The model under review builds one solid part; all positions refer to its coordinate system, in mm. A direction names the side the tool comes from. Coordinates: 2 decimals unless noted, no trailing zeros. Order: outer loops, then holes, each group sorted by start corner. A loop starts at its lowest first (then second) coordinate and runs counter-clockwise, first axis right, second up.
```python
from build123d import *

# Parameters (mm, degrees)
SKETCH1_W               = 28
SKETCH1_H               = 27
BOSS_EXTRUDE1_DEPTH     = 1.4
SKETCH2_R               = 1.55
CUT_EXTRUDE1_DEPTH      = 20.498974332
FILLET1_R               = 2
FILLET2_R               = 2
BOSS_EXTRUDE2_DEPTH     = 20
SKETCH5_W               = 14.5
SKETCH5_H               = 1
BOSS_EXTRUDE3_DEPTH     = 20
FILLET3_R               = 4
FILLET4_R               = 3
CUT_EXTRUDE2_DEPTH      = 32.957002439
CUT_EXTRUDE2_DEPTH_BACK = 32.957002439
FILLET6_R               = 2
FILLET7_R               = 3
SKETCH7_R               = 1.25
BOSS_EXTRUDE4_DEPTH     = 14.5
SKETCH8_R               = 6.5
BOSS_EXTRUDE5_DEPTH     = 5.5
FILLET8_R               = 1


with BuildPart() as part:
    # Sketch1 → Boss-Extrude1 (new body)
    with BuildSketch(Plane(origin=(0, 0, 0), x_dir=(1, 0, 0), z_dir=(0, 1, 0))):
        Rectangle(SKETCH1_W, SKETCH1_H)
    extrude(amount=BOSS_EXTRUDE1_DEPTH)

    # Sketch2 → Cut-Extrude1 (cut, through all)
    with BuildSketch(Plane(origin=(0, 1.4, 0), x_dir=(1, 0, 0), z_dir=(0, 1, 0))):
        with Locations(Location((-11, 10, 0), (0, 0, 270))):
            Circle(SKETCH2_R)
        with Locations(Location((-11, -10, 0), (0, 0, 270))):
            Circle(SKETCH2_R)
        with Locations(Location((11, -10, 0), (0, 0, 270))):
            Circle(SKETCH2_R)
        with Locations(Location((11, 10, 0), (0, 0, 270))):
            Circle(SKETCH2_R)
    extrude(amount=-CUT_EXTRUDE1_DEPTH, mode=Mode.SUBTRACT)

    # Fillet1
    fillet1_edges = [part.edges().sort_by_distance(p)[0] for p in [
        (-14, 0.7, -13.5),
        (14, 0.7, -13.5),
        (14, 0.7, 13.5),
        (-14, 0.7, 13.5),
    ]]
    fillet(fillet1_edges, radius=FILLET1_R)

    # Sketch3 → Revolve1 (revolve)
    with BuildSketch(Plane(origin=(0, 0, 0), x_dir=(0, 0, -1), z_dir=(1, 0, 0)), mode=Mode.PRIVATE) as revolve1_sk:
        Polygon((0, 0), (0, -4.5), (10, -4.5), (10, -2.033813378), (8.767949192, -1), (10.5, 0), align=None)
    revolve(revolve1_sk.sketch.rotate(Axis((0, 0, 0), (0, -1, 0)), 180), axis=Axis((0, 0, 0), (0, -1, 0)))

    # Fillet2
    fillet2_edges = [part.edges().sort_by_distance(p)[0] for p in [
        (0, -2.033813378, -10),
    ]]
    fillet(fillet2_edges, radius=FILLET2_R)

    # Sketch4 → Boss-Extrude2 (add)
    with BuildSketch(Plane.XZ.offset(4.5)):
        with BuildLine():
            Line((-7.25, 15), (-7.25, 6.887488657))
            ThreePointArc((-7.25, 6.887488657), (0, -10), (7.25, 6.887488657))
            Line((7.25, 6.887488657), (7.25, 15))
            Line((7.25, 15), (6.25, 15))
            Line((6.25, 15), (6.25, 6.475916923))
            ThreePointArc((6.25, 6.475916923), (0, -9), (-6.25, 6.475916923))
            Line((-6.25, 6.475916923), (-6.25, 15))
            Line((-6.25, 15), (-7.25, 15))
        make_face()
    extrude(amount=BOSS_EXTRUDE2_DEPTH)

    # Sketch5 → Boss-Extrude3 (add)
    with BuildSketch(Plane.XY.offset(15)):
        with Locations((0, -4)):
            Rectangle(SKETCH5_W, SKETCH5_H)
    extrude(amount=-BOSS_EXTRUDE3_DEPTH)

    # Fillet3
    fillet3_edges = [part.edges().sort_by_distance(p)[0] for p in [
        (6.25, -14.5, 6.475916923),
        (-6.25, -14.5, 6.475916923),
    ]]
    fillet(fillet3_edges, radius=FILLET3_R)

    # Fillet4
    fillet4_edges = [part.edges().sort_by_distance(p)[0] for p in [
        (-7.25, -14, 6.887488657),
        (7.25, -14, 6.887488657),
    ]]
    fillet(fillet4_edges, radius=FILLET4_R)

    # Sketch6 → Cut-Extrude2 (cut, two sides: drawn at the far end of the back side and taken through both)
    with BuildSketch(Plane(origin=(0, 0, 0), x_dir=(0, 0, -1), z_dir=(1, 0, 0)).offset(-CUT_EXTRUDE2_DEPTH_BACK)):
        with BuildLine():
            Line((10, -4.5), (7, -4.5))
            Line((7, -4.5), (-6.331273347, -18.89712301))
            ThreePointArc((-6.331273347, -18.89712301), (-11.824330937, -20.155299844), (-15, -15.5))
            Line((-15, -15.5), (-15, -24.5))
            Line((-15, -24.5), (10, -24.5))
            Line((10, -24.5), (10, -4.5))
        make_face()
    extrude(amount=CUT_EXTRUDE2_DEPTH + CUT_EXTRUDE2_DEPTH_BACK, mode=Mode.SUBTRACT)

    # Fillet6
    # the kernel refuses this fillet: 2 mm, written as the material it adds along each edge
    with BuildSketch(Plane(origin=(0, -4.5, 0), x_dir=(0.7884615384615388, 0, 0.6150840612199793), z_dir=(-0.6150840612199793, 0, 0.7884615384615388))) as fillet6_piece_1_section:
        with BuildLine():
            CenterArc((9 - FILLET6_R, -FILLET6_R), FILLET6_R, 0, 90)
            Line((9, -FILLET6_R), (9, 0))
            Line((9, 0), (9 - FILLET6_R, 0))
        make_face()
    fillet6_piece_1 = revolve(axis=Axis((0, -4.5, 0), (0, 1, 0)), revolution_arc=120.85908443, mode=Mode.PRIVATE)
    fillet6_piece_1 = split(fillet6_piece_1, bisect_by=Plane(origin=(7.790890129, -6.689454566, -4.972635416), z_dir=(0, 0.6794246019412827, 0.7337453306678888)), keep=Keep.TOP, mode=Mode.PRIVATE)
    add(fillet6_piece_1)
    with BuildSketch(Plane(origin=(-6.25, -4.5, 7.996092796), x_dir=(0, -1, 0), z_dir=(0, 0, 1))) as fillet6_piece_2:
        with BuildLine():
            CenterArc((FILLET6_R, FILLET6_R), FILLET6_R, 180, 90)
            Line((0, FILLET6_R), (0, 0))
            Line((0, 0), (FILLET6_R, 0))
        make_face()
    extrude(amount=7.003907204)
    with BuildSketch(Plane(origin=(10.25, -4.5, 7.996092796), x_dir=(-0.7884615384615388, 0, -0.6150840612199795), z_dir=(0.6150840612199795, 0, -0.7884615384615388))) as fillet6_piece_3:
        with BuildLine():
            CenterArc((4 + FILLET6_R, -FILLET6_R), FILLET6_R, 90, 90)
            Line((4, -FILLET6_R), (4, 0))
            Line((4, 0), (4 + FILLET6_R, 0))
        make_face()
    revolve(axis=Axis((10.25, -4.5, 7.996092796), (0, 1, 0)), revolution_arc=37.958028581)
    with BuildSketch(Plane(origin=(-10.25, -4.5, 7.996092796), x_dir=(1, 0, 0), z_dir=(0, 0, 1))) as fillet6_piece_4:
        with BuildLine():
            CenterArc((4 + FILLET6_R, -FILLET6_R), FILLET6_R, 90, 90)
            Line((4 + FILLET6_R, 0), (4, 0))
            Line((4, 0), (4, -FILLET6_R))
        make_face()
    revolve(axis=Axis((-10.25, -4.5, 7.996092796), (0, 1, 0)), revolution_arc=37.958028581)
    with BuildSketch(Plane(origin=(0, -4.5, 0), x_dir=(-0.12358318998339889, 0, -0.9923342154503829), z_dir=(0.9923342154503829, 0, -0.12358318998339889))) as fillet6_piece_5_section:
        with BuildLine():
            CenterArc((9 - FILLET6_R, -FILLET6_R), FILLET6_R, 360, 90)
            Line((9 - FILLET6_R, 0), (9, 0))
            Line((9, 0), (9, -FILLET6_R))
        make_face()
    fillet6_piece_5 = revolve(axis=Axis((0, -4.5, 0), (0, 1, 0)), revolution_arc=120.85908443, mode=Mode.PRIVATE)
    fillet6_piece_5 = split(fillet6_piece_5, bisect_by=Plane(origin=(-7.79089013, -6.689454565, -4.972635417), z_dir=(0, 0.6794246019412827, 0.7337453306678888)), keep=Keep.TOP, mode=Mode.PRIVATE)
    add(fillet6_piece_5)
    with BuildSketch(Plane(origin=(6.25, -4.5, 15), x_dir=(-1, 0, 0), z_dir=(0, 0, -1))) as fillet6_piece_6:
        with BuildLine():
            CenterArc((FILLET6_R, -FILLET6_R), FILLET6_R, 90, 90)
            Line((0, -FILLET6_R), (0, 0))
            Line((0, 0), (FILLET6_R, 0))
        make_face()
    extrude(amount=7.003907204)

    # Fillet7
    # the kernel refuses this fillet: 3 mm, written as the material it takes off along each edge
    with BuildSketch(Plane(origin=(7.25, -3.5, 22.5), x_dir=(-1, 0, 0), z_dir=(0, 0, -1))) as fillet7_piece_1_section:
        with BuildLine():
            CenterArc((FILLET7_R, -FILLET7_R), FILLET7_R, 90, 90)
            Line((0, -FILLET7_R), (0, 0))
            Line((0, 0), (FILLET7_R, 0))
        make_face()
    fillet7_piece_1 = extrude(amount=14.503907204, mode=Mode.PRIVATE)
    fillet7_piece_1 = fillet7_piece_1 - Plane(origin=(0, -4.174011866, 0), x_dir=(0, 0, 1), z_dir=(0, 1, 0)) * Cylinder(10, 42, mode=Mode.PRIVATE)
    add(fillet7_piece_1, mode=Mode.SUBTRACT)
    with BuildSketch(Plane(origin=(-7.25, -3.5, 22.5), x_dir=(0, -1, 0), z_dir=(0, 0, -1))) as fillet7_piece_2_section:
        with BuildLine():
            CenterArc((FILLET7_R, -FILLET7_R), FILLET7_R, 90, 90)
            Line((0, -FILLET7_R), (0, 0))
            Line((0, 0), (FILLET7_R, 0))
        make_face()
    fillet7_piece_2 = extrude(amount=14.503907204, mode=Mode.PRIVATE)
    fillet7_piece_2 = fillet7_piece_2 - Plane(origin=(0, -4.174011864, 0), x_dir=(0, 0, 1), z_dir=(0, 1, 0)) * Cylinder(10, 42, mode=Mode.PRIVATE)
    add(fillet7_piece_2, mode=Mode.SUBTRACT)
    with BuildSketch(Plane(origin=(10.25, -3.5, 7.996092796), x_dir=(0.999777856242507, 0, 0.021076958204088978), z_dir=(-0.021076958204088978, 0, 0.999777856242507))) as fillet7_piece_3_section:
        with BuildLine():
            CenterArc((3 + FILLET7_R, -FILLET7_R), FILLET7_R, 90, 90)
            Line((3, -FILLET7_R), (3, 0))
            Line((3, 0), (3 + FILLET7_R, 0))
        make_face()
    fillet7_piece_3 = revolve(axis=Axis((10.25, -3.5, 7.996092796), (0, 1, 0)), revolution_arc=181.20771018, mode=Mode.PRIVATE)
    fillet7_piece_3 = fillet7_piece_3 - Plane(origin=(0, -4.740784246, 0), x_dir=(0, 0, 1), z_dir=(0, 1, 0)) * Cylinder(10, 25, mode=Mode.PRIVATE)
    add(fillet7_piece_3, mode=Mode.SUBTRACT)
    with BuildSketch(Plane(origin=(-10.25, -3.5, 7.996092796), x_dir=(1, 0, 0), z_dir=(0, 0, 1))) as fillet7_piece_4_section:
        with BuildLine():
            CenterArc((3 + FILLET7_R, -FILLET7_R), FILLET7_R, 90, 90)
            Line((3, -FILLET7_R), (3, 0))
            Line((3, 0), (3 + FILLET7_R, 0))
        make_face()
    fillet7_piece_4 = revolve(axis=Axis((-10.25, -3.5, 7.996092796), (0, 1, 0)), revolution_arc=181.20771018, mode=Mode.PRIVATE)
    fillet7_piece_4 = fillet7_piece_4 - Plane(origin=(0, -4.344779192, 0), x_dir=(0, 0, 1), z_dir=(0, 1, 0)) * Cylinder(10, 24, mode=Mode.PRIVATE)
    add(fillet7_piece_4, mode=Mode.SUBTRACT)

    # Sketch7 → Boss-Extrude4 (add)
    with BuildSketch(Plane.ZY.offset(7.25)):
        with Locations((10, -15.5)):
            Circle(SKETCH7_R)
    extrude(amount=-BOSS_EXTRUDE4_DEPTH)

    # Sketch8 → Boss-Extrude5 (add, symmetric)
    with BuildSketch(Plane(origin=(0, 0, 0), x_dir=(0, 0, -1), z_dir=(1, 0, 0))):
        with Locations((-10, -15.5)):
            Circle(SKETCH8_R)
    extrude(amount=BOSS_EXTRUDE5_DEPTH, both=True)

    # Fillet8
    fillet8_edges = [part.edges().sort_by_distance(p)[0] for p in [
        (-5.5, -15.5, 16.5),
        (5.5, -15.5, 16.5),
    ]]
    fillet(fillet8_edges, radius=FILLET8_R)


solid = part.part
```
(1) Machinability: for faces 4 (the face through (6.824, -20.185, 11.746)), 5 (the face through (5.65, -5.07, 11.55)), 6 (the face through (0, -4.5, 3)), 7 (the face through (-8.6, -10.91, 2.66)), 8 (the face through (-6.39, -4.4, 11.55)), which of the approach directions +Z, -Z, +X, -X, +Y, -Y give a long, thin tool a straight path to every point of the face, cutting with its end or side? Answer none if there is none.
A:
face 4: +X, -Y
face 5: +Z
face 6: none
face 7: -Y
face 8: +Z, -X
(2) Draft analysis for pull direction X (two halves, no side actions). For faces 1 (the face through (0.063, -10.019, 6.506)), 2 (the face through (-7.418, -13.386, 7.007)), 3 (the face through (0, -4, 15)), state which applies: released by +X, released by -X, zero draft, split by the parting line, or undercut.
A:
face 1: undercut
face 2: released by -X
face 3: zero draft
(3) We need section C-C, the plane y = -17.5. Count the separate pieces of the cut face and the enclosed holes in it, and give its area (3 significant figures).
A:
separate pieces: 3
enclosed holes: 0
area: 155 mm2
(4) For pin 1 Ø3.5 at (x, y) = (2, -11.5) entering from +Z; pin 2 Ø6 at (y, z) = (-18, 9) entering from +X; pin 3 Ø2 at (y, z) = (-9.5, 2) entering from +X, all flat-tipped, find the tip position at first contact; note any pin that passes through.
A:
pin 1: stops at z = 16.1
pin 2: stops at x = 8
pin 3: stops at x = 9.95
(5) We need section A-A, the plane x = 11. Write out the cut boundary in (y, z), and give its area (3 significant figures).
A:
outline: (0, -13.5) - (1.4, -13.5) - (1.4, -11.55) - (0, -11.55) - close; (0, -8.45) - (1.4, -8.45) - (1.4, 8.45) - (0, 8.45) - close; (0, 11.55) - (1.4, 11.55) - (1.4, 13.5) - (0, 13.5) - close
area: 29.1 mm2
(6) Wall thickness on probe 1 along X at (y, z) = (1, 10); probe 2 along X at (y, z) = (-14, 7.25); probe 3 along Y at (x, z) = (11.75, 13): over which ranges is each line inside the solid? List them lowest first.
A:
probe 1: x = -14 to -12.55, -9.45 to 9.45, 12.55 to 14
probe 2: x = -7.34 to -6.32, -5.5 to 5.5, 6.32 to 7.34
probe 3: y = 0 to 1.4
(7) We need section B-B, the plane y = -6. Write out the cut boundary in (x, z), and give its area (3 significant figures).
A:
outline: (-8.28, -5.61) - (-6.96, -5.61) arc R8.94 cw to (-7.05, 5.5) arc R4.06 ccw to (-6.19, 8) - (-6.19, 15) - (-7.21, 15) - (-7.21, 8) arc R3.04 cw to (-7.61, 6.49) arc R10 ccw to start; (6.19, 8) arc R4.06 ccw to (7.05, 5.5) arc R8.94 cw to (6.96, -5.61) - (8.28, -5.61) arc R10 ccw to (7.61, 6.49) arc R3.04 cw to (7.21, 8) - (7.21, 15) - (6.19, 15) - close
area: 45.3 mm2
